Autodesk Inventor part; units mm, degrees
ref_plane "YZ Plane" through (0, 0, 0) normal (1, 0, 0) x (0, 1, 0)
ref_plane "XZ Plane" through (0, 0, 0) normal (0, 1, 0) x (-1, 0, 0)
ref_plane "XY Plane" through (0, 0, 0) normal (0, 0, 1) x (1, 0, 0)
sketch "Sketch1" plane through (0, 0, 0) normal (0, 1, 0) x (-1, 0, 0)
  line L0 (0, 0) -> (1, 0)
  line L1 (1, 0) -> (1, -6.5)
  line L2 (1, -6.5) -> (0, -6.5)
  line L3 (0, -6.5) -> (0, 0)
  line L4 (1, 0) -> (0, 0)
  line L5 (0, 0) -> (0, -1.6)
  line L6 (0, -1.6) -> (1, -1.6)
  line L7 (1, -1.6) -> (1, 0)
  line L8 (1, -1.6) -> (1.5, -1.6)
  line L9 (1.5, -1.6) -> (1.5, -2.6)
  line L10 (1.5, -2.6) -> (1, -2.6)
  line L11 (1, -2.6) -> (1, -1.6)
  line L12 (0, -1.6) -> (-0.5, -1.6)
  line L13 (-0.5, -1.6) -> (-0.5, -2.6)
  line L14 (-0.5, -2.6) -> (0, -2.6)
  line L15 (0, -2.6) -> (0, -1.6)
  dimension "d0" = 1
  dimension "d1" = 6.5
  dimension "d2" = 1.6
  dimension "d3" = 0.5
  dimension "d4" = 1
  dimension "d5" = 0.5
  dimension "d6" = 1
revolve "Revolution1" add sketch "Sketch1" angle 360 about axis through (0, 0, 0) along (-1, 0, 0) contours L6 L1 L2 L3 | L3 L14 L13 L12 | L8 L9 L10 L1
properties part number "idler_spacer"
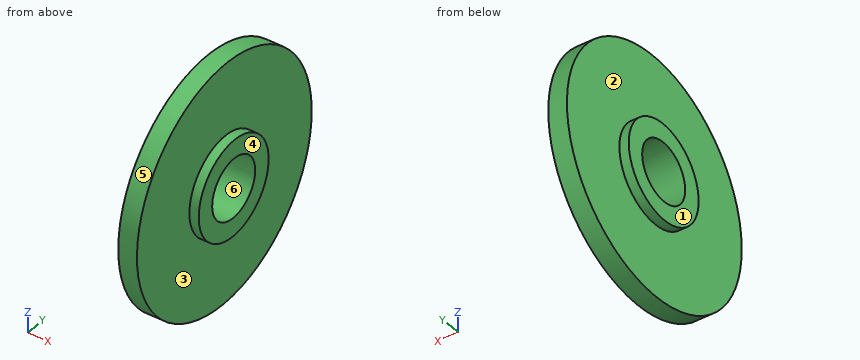
Geometry: final body of the model. Coordinates: model frame, mm. Face numbers are marked on the shaded views. A direction names the side the tool comes from. Give positions to 0.01 mm unless a question says otherwise; leave off trailing zeros. Order: outer loops, then holes, each group sorted by start corner. A loop starts at its lowest first (then second) coordinate and runs counter-clockwise, first axis right, second up. Notation, with made-up numbers: (67.5, 11.25) -> (87.5, 11.25) arc R27 ccw to (87.5, 34.25) -> close; hole circle Ø4 at (25, 42). An arc over 180 degrees is marked (long way). Answer as a JSON object with one key per item and string values.
Q1. Material intervals for probe 1 along Z at (x, y) = (-0.15, 0); probe 2 along X at (y, z) = (-4.25, -2), sorted ascending.
Entries:
{"probe 1": "z = -6.5 to -1.6, 1.6 to 6.5", "probe 2": "x = -1 to 0"}
Q2. Section D-D (z = 1.75). Output: boundary loops of the cut face in (x, y), plus the area to 3 significant figures.
Entries:
{"outline": "(-1.5, -1.92) -> (-1, -1.92) -> (-1, -6.26) -> (0, -6.26) -> (0, -1.92) -> (0.5, -1.92) -> (0.5, 1.92) -> (0, 1.92) -> (0, 6.26) -> (-1, 6.26) -> (-1, 1.92) -> (-1.5, 1.92) -> close", "area": "16.4 mm^2"}
Q3. Access query for the marked faces 1, 2 and 3. Directions: +Z, -Z, +X, -X, +Y, -Y. A direction counts if a zero-diameter tool reaches every point of the face in a straight line with its end or side. Return the directions, or none.
Entries:
{"face 1": "+Z, -Z, -X, +Y, -Y", "face 2": "-X", "face 3": "+X"}
Q4. Section C-C (x = -1.35). Output: boundary loops of the cut face in (y, z).
Entries:
{"outline": "circle Ø5.2 at (0, 0); hole circle Ø3.2 at (0, 0)"}
Q5. Draft query along Y for the marked faces 4, 5 and 6. Return one class per face: released by +Y, released by -Y, zero draft, split by the parting line, or undercut.
Entries:
{"face 4": "zero draft", "face 5": "split by the parting line", "face 6": "undercut"}
Q6. First-contact query: pin 1 (1 mm diameter, centred on x = -1, z = 4.5, fed in from +Y); pin 2 (1 mm diameter, centred on y = 1.5, z = -4.5, fed in from +X); pin 3 (6.5 mm diameter, centred on y = 0, z = -1.5, fed in from +X). Flat tips, straight axial feed; report the tip coordinate or a pass-through.
Entries:
{"pin 1": "stops at y = 5.12", "pin 2": "stops at x = 0", "pin 3": "stops at x = 0.5"}
Q7. Section A-A (y = 0). Output: boundary loops of the cut face in (x, z).
Entries:
{"outline": "(-1.5, -2.6) -> (-1, -2.6) -> (-1, -6.5) -> (0, -6.5) -> (0, -2.6) -> (0.5, -2.6) -> (0.5, -1.6) -> (-1.5, -1.6) -> close; (-1.5, 1.6) -> (0.5, 1.6) -> (0.5, 2.6) -> (0, 2.6) -> (0, 6.5) -> (-1, 6.5) -> (-1, 2.6) -> (-1.5, 2.6) -> close"}
